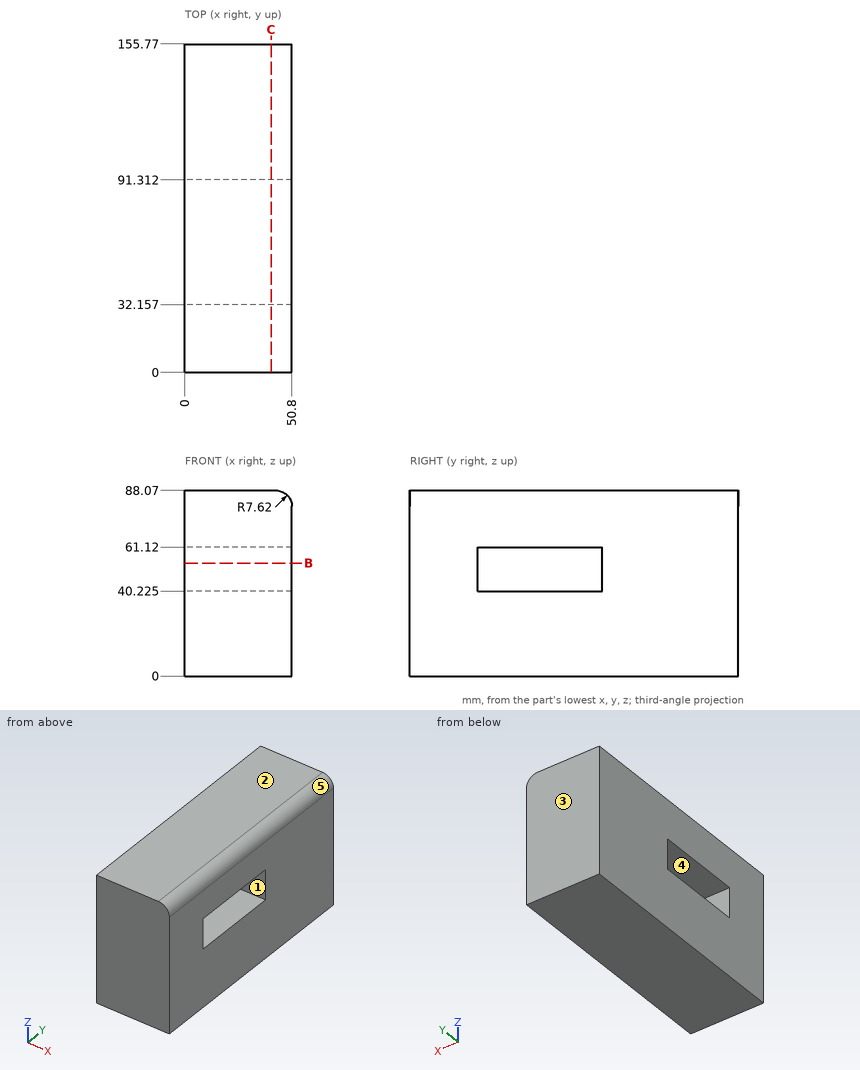
Could you check a few things on this drawing? It's one solid part, dimensions in mm from its lowest x, y, z. A direction names the side the tool comes from. Coordinates: 2 decimals unless noted, no trailing zeros. Write each loop counter-clockwise with the first axis right and the second up, starting at its lowest first coordinate (ties: lowest second). Pieces come first, ordered by that corner, then holes. Notation, with made-up numbers: (49, -21) - (74, -21) arc R4 ccw to (74, -14) - close; hole circle Ø5 at (-32.75, 40.5). An arc over 180 degrees is marked (long way). Use one line per item in the form item = value.
1) Suppose I cut it at B-B, the plane z = 53.5. Write out the boundary of the cut face in (x, y), plus the area to 3 significant figures.
Solved:
outline = (0, 0) - (50.8, 0) - (50.8, 32.16) - (0, 32.16) - close; (0, 91.31) - (50.8, 91.31) - (50.8, 155.77) - (0, 155.77) - close
area = 4,910 mm2
2) Suppose I cut it at C-C, the plane x = 41. Write out the boundary of the cut face in (y, z) (1 decimal).
Solved:
outline = (0, 0) - (155.8, 0) - (155.8, 88.1) - (0, 88.1) - close; hole (32.2, 40.2) - (91.3, 40.2) - (91.3, 61.1) - (32.2, 61.1) - close
3) On a 3-axis mill with a long thin cutter (end or side, diameter ignored), from which of +Z, -Z, +X, -X, +Y, -Y can I reach the whole of each face in a straight line? I mean the marked faces 1 and 2. Say none if no direction works.
Solved:
face_1 = +X, -X
face_2 = +Z, +X, -X, +Y, -Y
4) I need wall thicknesses on line 1 (Z direction, x = 37, y = 70) (1 decimal); line 2 (Y direction, x = 12.5, z = 59.5); line 3 (Z direction, x = 44, y = 90.5) (1 decimal). Which ranges of each line are inside material? Lowest first, please.
Solved:
line_1 = 0 to 40.2, 61.1 to 88.1
line_2 = 0 to 32.16, 91.31 to 155.77
line_3 = 0 to 40.2, 61.1 to 88
5) Thinking about a two-plate mould opening in Y: for the marked faces 3, 4 and 5, which applies, released by +Y, released by -Y, zero draft, split by the parting line, or undercut?
Solved:
face_3 = released by +Y
face_4 = undercut
face_5 = zero draft
